For this review, take the finished solid that the model builds, in its own axes (mm). A direction names the side the tool comes from. Coordinates: 2 decimals unless noted, no trailing zeros. Loops run counter-clockwise (first coordinate to the right, second up) from the corner with the lowest first, then second, coordinate; pieces in that order, holes last. Notation, with made-up numbers: (-8, -7.75) -> (41, -7.75) arc R18 ccw to (41, -2.75) -> close; hole circle Ø3 at (58.5, -29). An arc over 180 degrees is marked (long way). Answer in a Markdown table with one row per item.
from build123d import *

# Parameters (mm, degrees)
SKETCH1_W           = 800.1
SKETCH1_H           = 617.22
BOSS_EXTRUDE1_DEPTH = 304.8
SKETCH3_W           = 800.1
SKETCH3_H           = 617.22
SKETCH3_W_2         = 578.099229306
SKETCH3_H_2         = 562.360466338
CUT_EXTRUDE1_DEPTH  = 177.8
SKETCH5_W           = 578.099229306
SKETCH5_H           = 127
CUT_EXTRUDE3_DEPTH  = 776.110031957
SKETCH6_W           = 381
SKETCH6_H           = 324.666103145
CUT_EXTRUDE4_DEPTH  = 536.623911527


with BuildPart() as part:
    # Sketch1 → Boss-Extrude1 (new body)
    with BuildSketch(Plane(origin=(0, 0, 0), x_dir=(1, 0, 0), z_dir=(0, 1, 0))):
        Rectangle(SKETCH1_W, SKETCH1_H)
    extrude(amount=-BOSS_EXTRUDE1_DEPTH)

    # Sketch3 → Cut-Extrude1 (cut)
    with BuildSketch(Plane.XZ.offset(304.8)):
        Rectangle(SKETCH3_W, SKETCH3_H)
        Rectangle(SKETCH3_W_2, SKETCH3_H_2, mode=Mode.SUBTRACT)
    extrude(amount=-CUT_EXTRUDE1_DEPTH, mode=Mode.SUBTRACT)

    # Sketch5 → Cut-Extrude3 (cut, through all)
    with BuildSketch(Plane.XY.offset(281.180233169)):
        with Locations((0, -241.3)):
            Rectangle(SKETCH5_W, SKETCH5_H)
    extrude(amount=-CUT_EXTRUDE3_DEPTH, mode=Mode.SUBTRACT)

    # Sketch6 → Cut-Extrude4 (cut, through all)
    with BuildSketch(Plane(origin=(0, 0, 0), x_dir=(1, 0, 0), z_dir=(0, 1, 0))):
        with Locations((0, 146.276948428)):
            Rectangle(SKETCH6_W, SKETCH6_H)
    extrude(amount=-CUT_EXTRUDE4_DEPTH, mode=Mode.SUBTRACT)


solid = part.part
Item 1: Take a section at A-A, the plane z = -83.5. State the section outline as (x, y) points.
Worked answers:
| item | result |
|---|---|
| outline | (-400.05, -127) -> (-289.05, -127) -> (-289.05, -177.8) -> (-190.5, -177.8) -> (-190.5, 0) -> (-400.05, 0) -> close; (190.5, -177.8) -> (289.05, -177.8) -> (289.05, -127) -> (400.05, -127) -> (400.05, 0) -> (190.5, 0) -> close |
Item 2: For L1, parallel to X at y = -85, z = -269.5; L2, parallel to Z at x = -173, y = -89; L3, parallel to X at y = -158, z = -187.5, list the stretches that pass through material, from the lowest coordinate up.
Worked answers:
| item | result |
|---|---|
| L1 | -400.05 to -190.5, 190.5 to 400.05 |
| L2 | 16.06 to 308.61 |
| L3 | -289.05 to -190.5, 190.5 to 289.05 |
Item 3: Take a section at B-B, the plane y = -46.5. State the section outline as (x, z) points.
Worked answers:
| item | result |
|---|---|
| outline | (-400.05, -308.61) -> (-190.5, -308.61) -> (-190.5, 16.06) -> (190.5, 16.06) -> (190.5, -308.61) -> (400.05, -308.61) -> (400.05, 308.61) -> (-400.05, 308.61) -> close |
Item 4: The part is to be moulded in two halves that separate along X. For faces 6 (the flat face through (-6, 0, 64)), 7 (the flat face through (-3, -88, 16.056)), 8 (the flat face through (-190.5, -88, -144)), 9 (the flat face through (-289.05, -153, -4)), say which applies: +X half, -X half, draft (parallel to the pull), parting line (faces both ways), or undercut.
Worked answers:
| item | result |
|---|---|
| face 6 | draft |
| face 7 | undercut |
| face 8 | undercut |
| face 9 | -X half |
Item 5: Take a section at D-D, the plane x = -113. State the section outline as (y, z) points, and give its area (3 significant figures).
Worked answers:
| item | result |
|---|---|
| outline | (-177.8, 16.06) -> (0, 16.06) -> (0, 308.61) -> (-127, 308.61) -> (-127, 281.18) -> (-177.8, 281.18) -> close |
| area | 50,600 mm² |
Item 6: Take a section at C-C, the plane x = -239.5. State the section outline as (y, z) points, and give its area (3 significant figures).
Worked answers:
| item | result |
|---|---|
| outline | (-177.8, -281.18) -> (-127, -281.18) -> (-127, -308.61) -> (0, -308.61) -> (0, 308.61) -> (-127, 308.61) -> (-127, 281.18) -> (-177.8, 281.18) -> close |
| area | 107,000 mm² |
Item 7: For faces 1 (the flat face through (-240, -153, -281.18)), 2 (the flat face through (-4, -177.8, 66)), 3 (the flat face through (-4, -153, 281.18)), 4 (the flat face through (190.5, -88, -144)), 5 (the flat face through (289.05, -153, -4)), list the 3-axis set-ups (+Z, -Z, +X, -X, +Y, -Y) from which the entire face can be reached by the end or side of a thin tool; tool diameter is ignored.
Worked answers:
| item | result |
|---|---|
| face 1 | -Z, +X, -X, -Y |
| face 2 | +Z, -Z, +X, -X, -Y |
| face 3 | +Z, +X, -X, -Y |
| face 4 | -Z, +Y, -Y |
| face 5 | +Z, -Z, +X, -Y |
Item 8: Insertion check: pin 1 (8 mm diameter, centred on y = -148.5, z = -66.5, fed in from +X); pin 2 (4 mm diameter, centred on x = 5.5, y = -98, fed in from -Z); pin 3 (15 mm diameter, centred on y = -143, z = -106, fed in from -X). Each pin has a flat end and moves straight along its axis. Give the tip position at first contact, or say it passes through.
Worked answers:
| item | result |
|---|---|
| pin 1 | x = 289.05 |
| pin 2 | z = 16.06 |
| pin 3 | x = -289.05 |
